Work out the finished part from the listing and answer in its coordinate system (mm). A direction names the side the tool comes from. Round coordinates to 2 decimals unless told otherwise and drop trailing zeros. Write each loop counter-clockwise with the first axis right and the second up, starting at its lowest first coordinate (ties: lowest second). Pieces come first, ordered by that corner, then holes. Notation, with made-up numbers: (-34.5, 23) - (21.5, 23) arc R20 ccw to (21.5, 56) - close; hole circle Ø7 at (-33, 25.5). An arc over 180 degrees is marked (long way). Write item = value, one per line. Start each with the question number.
from build123d import *

# Parameters (mm, degrees)
SKETCH18_R           = 31.5
BOSS_EXTRUDE13_DEPTH = 16
SKETCH19_R           = 2
BOSS_EXTRUDE14_DEPTH = 2


with BuildPart() as part:
    # Sketch18 → Boss-Extrude13 (new body)
    with BuildSketch(Plane(origin=(0, 0, 0), x_dir=(1, 0, 0), z_dir=(0, 1, 0))):
        with BuildLine():
            Line((-39.5, 0), (-39.5, 42.5))
            Line((-39.5, 42.5), (39.5, 42.5))
            Line((39.5, 42.5), (39.5, 0))
            ThreePointArc((39.5, 0), (0, -39.5), (-39.5, 0))
        make_face()
        Circle(SKETCH18_R, mode=Mode.SUBTRACT)
    extrude(amount=BOSS_EXTRUDE13_DEPTH)

    # Sketch19 → Boss-Extrude14 (add)
    with BuildSketch(Plane.XZ):
        with Locations((-35.5, -38.5)):
            Circle(SKETCH19_R)
        with Locations((35.5, -38.5)):
            Circle(SKETCH19_R)
    extrude(amount=BOSS_EXTRUDE14_DEPTH)


solid = part.part
1. Consider line 1 (Z direction, x = 0, y = 10); line 2 (X direction, y = 1, z = -5); line 3 (Y direction, x = 28, z = 17.5). Determine where each line is inside the solid, lowest interval first.
2. Find section B-B on y = 5.5. Give the vertices of the cut face in (x, z), plus the area to 3 significant figures.
3. Find section D-D on z = -38.5. Give the vertices of the cut face in (x, y).
4. Find section C-C on x = 18. Give the vertices of the cut face in (y, z).
5. Which of the six approach directions +Z, -Z, +X, -X, +Y, -Y give full straight-line access (tool end or side, diameter ignored) to faces 4 (the face through (36.423, -0.986, -40.274)), 5 (the face through (18, 16, -29))?
6. Find section A-A on z = -18. Give the vertices of the cut face in (x, y).
7. For a pull along X with two mould halves and no side action, classify faces 1 (the face through (-34.577, -0.986, -40.274)), 2 (the face through (-36, -2, -38)), 3 (the face through (39.5, 8, -22)) as released by +X, released by -X, zero draft, split by the parting line, or undercut.
8. Each of these flat-tipped pins is pushed along its axis until it touches: pin 1 (4 mm diameter, centred on y = 7, z = 0.5, fed in from -X); pin 2 (10 mm diameter, centred on x = 8.5, y = 5, fed in from +Z); pin 3 (1 mm diameter, centred on x = 1.5, y = 10, fed in from +Z); pin 4 (1 mm diameter, centred on x = -27.5, y = 6.5, fed in from +Z). Where does it stop, or does it pass through?
Answer key:
q1.line_1 = -42.5 to -31.5, 31.5 to 39.5
q1.line_2 = -39.5 to -31.1, 31.1 to 39.5
q1.line_3 = 0 to 16
q2.outline = (-39.5, -42.5) - (39.5, -42.5) - (39.5, 0) arc R39.5 ccw to (-39.5, 0) - close; hole circle Ø63 at (0, 0)
q2.area = 2,690 mm²
q3.outline = (-39.5, 0) - (-37.5, 0) - (-37.5, -2) - (-33.5, -2) - (-33.5, 0) - (33.5, 0) - (33.5, -2) - (37.5, -2) - (37.5, 0) - (39.5, 0) - (39.5, 16) - (-39.5, 16) - close
q4.outline = (0, -42.5) - (16, -42.5) - (16, -25.85) - (0, -25.85) - close; (0, 25.85) - (16, 25.85) - (16, 35.16) - (0, 35.16) - close
q5.face_4 = -Y
q5.face_5 = +Z, -Z, +X, -X, +Y
q6.outline = (-39.5, 0) - (-25.85, 0) - (-25.85, 16) - (-39.5, 16) - close; (25.85, 0) - (39.5, 0) - (39.5, 16) - (25.85, 16) - close
q7.face_1 = undercut
q7.face_2 = zero draft
q7.face_3 = released by +X
q8.pin_1 = -39.5
q8.pin_2 = 39.34
q8.pin_3 = 39.49
q8.pin_4 = 28.83
